from build123d import *

# Parameters (mm, degrees)
F0_R     = 2.5
F1_DEPTH = 15
F3_R     = 1.5
F4_DEPTH = 5


# Not quite as in the source:
# - a fillet or chamfer that OpenCascade refuses, or shapes differently, is made with other operations: its cross-section is extruded or revolved along the edge and cut away or added


with BuildPart() as f1:
    # F0 (on Top) → F1 (new body)
    with BuildSketch(Plane.XY):
        Polygon((-5, 10), (-15, 10), (-15, 5), (-15, -10), (15, -10), (15, 10), align=None)
        with Locations((-10, -5)):
            Circle(F0_R, mode=Mode.SUBTRACT)
        with Locations((10, -5)):
            Circle(F0_R, mode=Mode.SUBTRACT)
        with BuildLine():
            ThreePointArc((-7.5, 5), (-10, 2.5), (-12.5, 5))
            ThreePointArc((-12.5, 5), (-10, 7.5), (-7.5, 5))
        make_face(mode=Mode.SUBTRACT)
        Circle(F0_R, mode=Mode.SUBTRACT)
        with Locations((10, 5)):
            Circle(F0_R, mode=Mode.SUBTRACT)
    extrude(amount=F1_DEPTH)

    # F2: chamfer of 3 on 5 edges, made by hand

    # F2_s1 → F2_t2 (revolve, cut)
    with BuildSketch(Plane.XZ.offset(-5)):
        Polygon((-4.5, 15), (-7.5, 12), (-7.5, 15), align=None)
    revolve(axis=Axis((-10, 5, 15), (0, 0, 1)), mode=Mode.SUBTRACT)

    # F2_s3 → F2_t4 (revolve, cut)
    with BuildSketch(Plane.XZ):
        Polygon((5.5, 15), (2.5, 12), (2.5, 15), align=None)
    revolve(axis=Axis((0, 0, 15), (0, 0, 1)), mode=Mode.SUBTRACT)

    # F2_s5 → F2_t6 (revolve, cut)
    with BuildSketch(Plane.XZ.offset(5)):
        Polygon((-4.5, 15), (-7.5, 12), (-7.5, 15), align=None)
    revolve(axis=Axis((-10, -5, 15), (0, 0, 1)), mode=Mode.SUBTRACT)

    # F2_s7 → F2_t8 (revolve, cut)
    with BuildSketch(Plane.XZ.offset(-5)):
        Polygon((15.5, 15), (12.5, 12), (12.5, 15), align=None)
    revolve(axis=Axis((10, 5, 15), (0, 0, 1)), mode=Mode.SUBTRACT)

    # F2_s9 → F2_t10 (revolve, cut)
    with BuildSketch(Plane.XZ.offset(5)):
        Polygon((15.5, 15), (12.5, 12), (12.5, 15), align=None)
    revolve(axis=Axis((10, -5, 15), (0, 0, 1)), mode=Mode.SUBTRACT)

    # F3 (on face) → F4 (cut)
    with BuildSketch(Plane(origin=(-15, 0, 0), x_dir=(0, -1, 0), z_dir=(-1, 0, 0))):
        with Locations((0, 7.5)):
            Circle(F3_R)
        with Locations((-5, 11.2557266839)):
            Circle(F3_R)
        with Locations((-5, 3.7442733161)):
            Circle(F3_R)
        with Locations((5, 11.2557266839)):
            Circle(F3_R)
        with Locations((5, 3.7442733161)):
            Circle(F3_R)
    extrude(amount=-F4_DEPTH, mode=Mode.SUBTRACT)


solid = f1.part
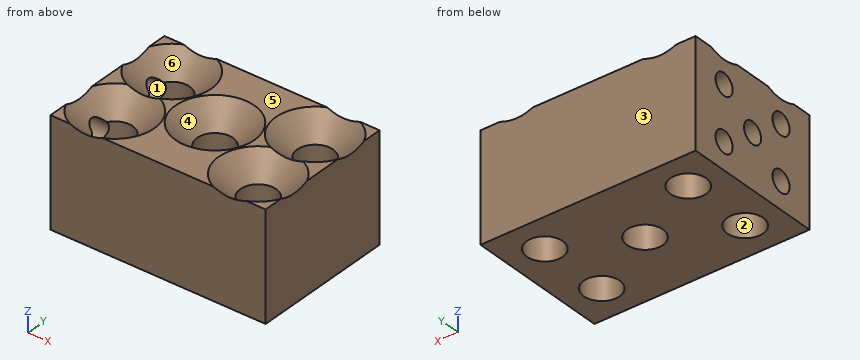
The model under review builds one solid part; all positions refer to its coordinate system, in mm. Face numbers are marked on the shaded views. A direction names the side the tool comes from. Round coordinates to 2 decimals unless told otherwise and drop trailing zeros. Loops run counter-clockwise (first coordinate to the right, second up) from the corner with the lowest first, then second, coordinate; pieces in that order, holes last. Notation, with made-up numbers: (8, 6.25) -> (49, 6.25) arc R13 ccw to (49, 16.25) -> close; hole circle Ø4 at (66, 12.25). An arc over 180 degrees is marked (long way). Return JSON: item names as keys, results as strings.
(1) For pin 1 (8 mm diameter, centred on x = 10, y = -5, fed in from +Z); pin 2 (4 mm diameter, centred on x = -6.5, y = -2, fed in from -Z); pin 3 (6 mm diameter, centred on x = 0, y = 0, fed in from +Z); pin 4 (1.5 mm diameter, centred on y = -0.5, z = 8, fed in from -X), all flat-tipped, find the tip position at first contact; note any pin that passes through.
Solved:
{"pin 1": "z = 13.5", "pin 2": "z = 0", "pin 3": "z = 12.5", "pin 4": "x = -10"}
(2) Add section C-C on x = 0. Write out the cut boundary in (y, z), plus the area to 3 significant figures.
Solved:
{"outline": "(-10, 0) -> (-2.5, 0) -> (-2.5, 12) -> (-5.5, 15) -> (-10, 15) -> close; (2.5, 0) -> (10, 0) -> (10, 15) -> (5.5, 15) -> (2.5, 12) -> close", "area": "216 mm2"}
(3) Add section B-B on z = 13.75. Write out the cut boundary in (x, y).
Solved:
{"outline": "(-15, -10) -> (15, -10) -> (15, 10) -> (-15, 10) -> close; hole circle Ø8.5 at (-10, -5); hole circle Ø8.5 at (-10, 5); hole circle Ø8.5 at (0, 0); hole circle Ø8.5 at (10, -5); hole circle Ø8.5 at (10, 5)"}
(4) The part is to be moulded in two halves that separate along Y. For the marked faces 3, 4, 5 and 6, say which applies: released by +Y, released by -Y, zero draft, split by the parting line, or undercut.
Solved:
{"face 3": "released by +Y", "face 4": "undercut", "face 5": "zero draft", "face 6": "undercut"}
(5) For line 1 (Y direction, x = -10, z = 5); line 2 (X direction, y = 3.25, z = 10); line 3 (Z direction, x = -12.7, y = -5), list the stretches that pass through material, from the lowest coordinate up.
Solved:
{"line 1": "-10 to -7.5, -2.5 to 2.5, 7.5 to 10", "line 2": "-15 to -11.79, -8.21 to 8.21, 11.79 to 15", "line 3": "0 to 2.24, 5.24 to 9.76"}
(6) Add section A-A on x = 10. Write out the cut boundary in (y, z), plus the area to 4 significant figures.
Solved:
{"outline": "(-10, 0) -> (-7.5, 0) -> (-7.5, 12) -> (-10, 14.5) -> close; (-2.5, 0) -> (2.5, 0) -> (2.5, 12) -> (0, 14.5) -> (-2.5, 12) -> close; (7.5, 0) -> (10, 0) -> (10, 14.5) -> (7.5, 12) -> close", "area": "132.5 mm2"}
(7) For the marked faces 1 and 2, list the 3-axis set-ups (+Z, -Z, +X, -X, +Y, -Y) from which the entire face can be reached by the end or side of a thin tool; tool diameter is ignored.
Solved:
{"face 1": "-X", "face 2": "+Z, -Z"}
(8) Add section D-D on z = 10.5. Write out the cut boundary in (x, y).
Solved:
{"outline": "(-15, -10) -> (15, -10) -> (15, 10) -> (-15, 10) -> (-15, 6.3) -> (-12.14, 6.3) arc R2.5 cw (long way) to (-12.14, 3.7) -> (-15, 3.7) -> (-15, -3.7) -> (-12.14, -3.7) arc R2.5 cw (long way) to (-12.14, -6.3) -> (-15, -6.3) -> close; hole circle Ø5 at (0, 0); hole circle Ø5 at (10, -5); hole circle Ø5 at (10, 5)"}
